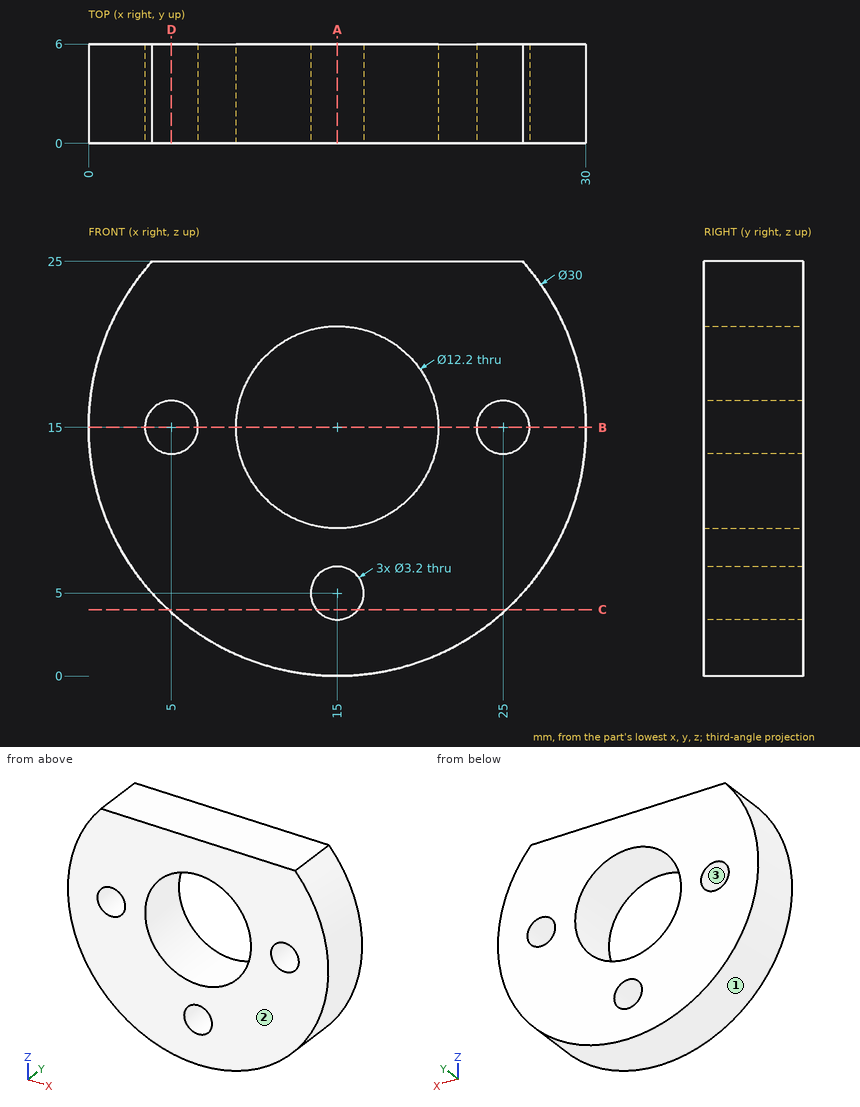
Input: dimensioned drawing with shaded views. Units: mm. Origin: part minimum x, y, z. Round coordinates to 2 decimals unless told otherwise and drop trailing zeros. Loops run counter-clockwise (first coordinate to the right, second up) from the corner with the lowest first, then second, coordinate; pieces in that order, holes last. Notation, with made-up numbers: M 15.5,70 L 61.5,70 A16 ccw 61.5,75 Z; hole C 50,-40 d2. An arc over 180 degrees is marked long. One line per question, with ' | ' between items.
(1) Pull-direction query (Z, two-part tool) for the marked faces 1, 2 and 3; classes: +Z half, -Z half, draft (parallel to the pull), parting line (faces both ways), or undercut.
Check result:
face 1: parting line | face 2: draft | face 3: undercut
(2) Contact query for flat-ended pins moving along their axis: P1, Ø1, axis at x = 11, y = 5, coming from the -Z side; P2, Ø1.5, axis at x = 16, y = 5, coming from the -Z side; P3, Ø1.9, axis at x = 5, z = 15, coming from the +Y side; P4, Ø1.5, axis at y = 1, z = 5.5, coming from the -X side. Output: stop coordinate, or through.
Check result:
P1: stops at z = 0.41 | P2: stops at z = 0 | P3: passes through | P4: stops at x = 2.82
(3) Cut plane C-C on z = 4. Return the cut outline in (x, y).
Check result:
outline: M 4.8,0 L 13.75,0 L 13.75,6 L 4.8,6 Z; M 16.25,0 L 25.2,0 L 25.2,6 L 16.25,6 Z
(4) Cut plane B-B on z = 15. Return the cut outline in (x, y).
Check result:
outline: M 0,0 L 3.4,0 L 3.4,6 L 0,6 Z; M 6.6,0 L 8.9,0 L 8.9,6 L 6.6,6 Z; M 21.1,0 L 23.4,0 L 23.4,6 L 21.1,6 Z; M 26.6,0 L 30,0 L 30,6 L 26.6,6 Z
(5) Cut plane A-A on x = 15. Return the cut outline in (y, z), plus the area to 3 significant figures.
Check result:
outline: M 0,0 L 6,0 L 6,3.4 L 0,3.4 Z; M 0,6.6 L 6,6.6 L 6,8.9 L 0,8.9 Z; M 0,21.1 L 6,21.1 L 6,25 L 0,25 Z | area: 57.6 mm2
(6) Material intervals for line 1 along Z through (x, y) = (15, 3.4); line 2 along Z through (x, y) = (14, 4.6); line 3 along Z through (x, y) = (5, 3.9), sorted ascending. Write a range as from..to.
Check result:
line 1: z = 0..3.4, 6.6..8.9, 21.1..25 | line 2: z = 0.03..3.75, 6.25..8.98, 21.02..25 | line 3: z = 3.82..13.4, 16.6..25
(7) Cut plane D-D on x = 5. Return the cut outline in (y, z).
Check result:
outline: M 0,3.82 L 6,3.82 L 6,13.4 L 0,13.4 Z; M 0,16.6 L 6,16.6 L 6,25 L 0,25 Z
